Read the model definition and answer for the solid it produces. Units are mm, in the model's axes. Face numbers are marked on the shaded views. A direction names the side the tool comes from. Coordinates: 2 decimals unless noted, no trailing zeros. Write each loop counter-clockwise with the first axis right and the second up, starting at its lowest first coordinate (ties: lowest second). Pieces come first, ordered by that corner, then holes. Notation, with made-up numbers: (27.5, 15) -> (68.5, 15) arc R25 cw to (68.5, 47) -> close; hole circle Ø3 at (-35.5, 77). An arc over 180 degrees is marked (long way). One line per item, written item: value. Start each with the question number.
1. Find section C-C, the plane y = 4.75. Write down the section's boundary in (x, z), and give its area (3 significant figures).
2. Consider line 1 along X through (y, z) = (22.5, 0); line 2 along Y through (x, z) = (4.5, 22); line 3 along Y through (x, z) = (15.5, -2.5). Determine where each line is inside the solid, lowest interval first.
3. For a pull along X with two mould halves and no side action, classify the marked faces 4, 5 and 6 as pulls with the +X half, pulls with the -X half, needs draft (parallel to the pull), parting line crosses it, or undercut.
4. Given P1, Ø6, axis at x = 2.5, y = 11.5, coming from the -Z side; P2, Ø6, axis at x = 14.5, z = 18.5, coming from the -Y side; P3, Ø16, axis at x = -10.5, z = -12, coming from the +Y side, each flat-ended and moving along its own axis, determine where each tip first touches the part or whether it passes through.
5. Find section A-A, the plane z = 0. Write down the section's boundary in (x, y), and give its area (3 significant figures).
6. Find section B-B, the plane y = 12. Write down the section's boundary in (x, z), and give its area (3 significant figures).
7. For the marked faces 1, 2 and 3, determine the directions among +Z, -Z, +X, -X, +Y, -Y from which every point of the face is accessible in a straight line to the end or side of a thin tool.
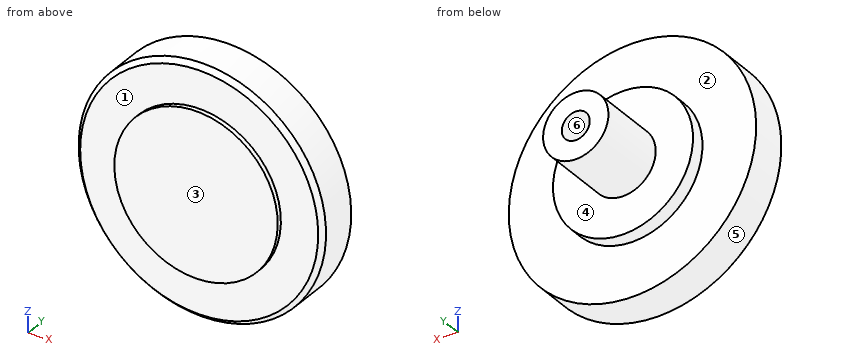
```python
from build123d import *

# Parameters (mm, degrees)
CROQUIS2_R              = 26.5
SALIENTE_EXTRUIR1_DEPTH = 8
CROQUIS3_R              = 26.5
SALIENTE_EXTRUIR2_DEPTH = 1
SALIENTE_EXTRUIR2_TAPER = 45
CROQUIS4_R              = 17.5
SALIENTE_EXTRUIR3_DEPTH = 1
CROQUIS5_R              = 15
SALIENTE_EXTRUIR4_DEPTH = 3
CROQUIS6_R              = 7
SALIENTE_EXTRUIR5_DEPTH = 15
CROQUIS7_R              = 3
CORTAR_EXTRUIR1_DEPTH   = 9


with BuildPart() as part:
    # Croquis2 → Saliente-Extruir1 (new body)
    with BuildSketch(Plane(origin=(0, 0, 0), x_dir=(1, 0, 0), z_dir=(0, 1, 0))):
        with Locations(Location((0, 0, 0), (0, 0, 270))):
            Circle(CROQUIS2_R)
    extrude(amount=SALIENTE_EXTRUIR1_DEPTH)

    # Croquis3 → Saliente-Extruir2 (add)
    with BuildSketch(Plane(origin=(0, 0, 0), x_dir=(-1, 0, 0), z_dir=(0, -1, 0))):
        with Locations(Location((0, 0, 0), (0, 0, 90))):
            Circle(CROQUIS3_R)
    extrude(amount=SALIENTE_EXTRUIR2_DEPTH, taper=SALIENTE_EXTRUIR2_TAPER)

    # Croquis4 → Saliente-Extruir3 (add)
    with BuildSketch(Plane(origin=(0, -1, 0), x_dir=(-1, 0, 0), z_dir=(0, -1, 0))):
        with Locations(Location((0, 0, 0), (0, 0, 90))):
            Circle(CROQUIS4_R)
    extrude(amount=SALIENTE_EXTRUIR3_DEPTH)

    # Croquis5 → Saliente-Extruir4 (add)
    with BuildSketch(Plane(origin=(0, 8, 0), x_dir=(1, 0, 0), z_dir=(0, 1, 0))):
        with Locations(Location((0, 0, 0), (0, 0, 270))):
            Circle(CROQUIS5_R)
    extrude(amount=SALIENTE_EXTRUIR4_DEPTH)

    # Croquis6 → Saliente-Extruir5 (add)
    with BuildSketch(Plane(origin=(0, 11, 0), x_dir=(1, 0, 0), z_dir=(0, 1, 0))):
        with Locations(Location((0, 0, 0), (0, 0, 270))):
            Circle(CROQUIS6_R)
    extrude(amount=SALIENTE_EXTRUIR5_DEPTH)

    # Croquis7 → Cortar-Extruir1 (cut)
    with BuildSketch(Plane(origin=(0, 26, 0), x_dir=(1, 0, 0), z_dir=(0, 1, 0))):
        with Locations(Location((0, 0, 0), (0, 0, 270))):
            Circle(CROQUIS7_R)
    extrude(amount=-CORTAR_EXTRUIR1_DEPTH, mode=Mode.SUBTRACT)


solid = part.part
```
Answer block:
1. outline: circle Ø53 at (0, 0)
1. area: 2,210 mm2
2. line 1: x = -7 to -3, 3 to 7
2. line 2: y = -1 to 8
2. line 3: y = -2 to 8
3. face 4: needs draft
3. face 5: parting line crosses it
3. face 6: undercut
4. P1: stops at z = -15
4. P2: stops at y = -1
4. P3: stops at y = 11
5. outline: (-26.5, 0) -> (-25.5, -1) -> (-17.5, -1) -> (-17.5, -2) -> (17.5, -2) -> (17.5, -1) -> (25.5, -1) -> (26.5, 0) -> (26.5, 8) -> (15, 8) -> (15, 11) -> (7, 11) -> (7, 26) -> (3, 26) -> (3, 17) -> (-3, 17) -> (-3, 26) -> (-7, 26) -> (-7, 11) -> (-15, 11) -> (-15, 8) -> (-26.5, 8) -> close
5. area: 757 mm2
6. outline: circle Ø14 at (0, 0)
6. area: 154 mm2
7. face 1: -Y
7. face 2: +Y
7. face 3: +Z, -Z, +X, -X, -Y
